Can you work these out from the model? Positions are in its coordinate system, mm. A direction names the side the tool comes from. Coordinates: 2 decimals unless noted, no trailing zeros. Use a Markdown table: item, result. Add a question column.
(1) If I drill on L1, parallel to X at y = -8, z = 11.9; L2, parallel to X at y = -8, z = 11.95; L3, parallel to Y at x = 17, z = 9.25, over which ranges is the centre line in solid material (lowest first)? Write a range as [from, to].
(2) On a 3-axis mill with a long thin cutter (end or side, diameter ignored), from which of +Z, -Z, +X, -X, +Y, -Y can I reach the whole of each face in a straight line? I mean faces 1 (the flat face through (21.38, -5.16, 7.04)), 2 (the flat face through (13, -18, 2)). Say none if no direction works.
(3) We'd pull the mould along X, two halves only. Please class faces 3 (the conical face through (32.351, -32.649, 1.877)), 4 (the cylindrical face through (8.77, 3.44, 6.94)), 5 (the flat face through (20.4, -4.4, 4)), 6 (the flat face through (20.4, -4.4, 10)): pulls with the +X half, pulls with the -X half, needs draft (parallel to the pull), parting line crosses it, or undercut.
(4) I want a section at A-A (z = 9.25). State how many separate pieces and enclosed holes the cut face has, and give its area (3 significant figures).
(5) For pin 1 Ø9.5 at (x, y) = (19, -3) entering from -Z; pin 2 Ø5 at (x, y) = (38.5, -19.5) entering from +Z; pin 3 Ø1 at (y, z) = (-16.5, 9.5) entering from +X; pin 4 Ø7 at (x, y) = (22.5, -12.5) entering from +Z, each with a flat end and sliding along its axis, tell me the tip position at first contact or that it passes through.
```python
from build123d import *

# Parameters (mm, degrees)
BOSS_EXTRUDE1_DEPTH         = 2
BOSS_EXTRUDE2_DEPTH         = 1
CHAMFER1_SIZE               = 0.25
BOSS_EXTRUDE3_DEPTH         = 8
CUT_EXTRUDE_THIN1_START     = -11.887644895
CUT_EXTRUDE_THIN1_OUTLINE_W = 0.5
CUT_EXTRUDE_THIN1_OUTLINE_H = 6
CUT_EXTRUDE_THIN1_DEPTH     = 23
CUT_EXTRUDE1_START          = -0.2
CUT_EXTRUDE1_DEPTH          = 0.2
FILLET1_R                   = 0.1


# Read off the part's stored shape, not the designer's step: Cut-Extrude-Thin1
with BuildPart() as part:
    # Sketch1 → Boss-Extrude1 (new body)
    with BuildSketch(Plane.XY):
        with BuildLine():
            Line((0.767949192, 12), (0.767949192, -48))
            ThreePointArc((0.767949192, -48), (32.790806806, -32.362304412), (45.75, 0.834988321))
            Line((45.75, 0.834988321), (45.75, 12))
            Line((45.75, 12), (0.767949192, 12))
        make_face()
    extrude(amount=BOSS_EXTRUDE1_DEPTH)

    # Sketch2 → Boss-Extrude2 (add)
    with BuildSketch(Plane.XY.offset(2)):
        with BuildLine():
            Line((8.80088089, -1.616278944), (12.994920502, -4.6656628))
            ThreePointArc((12.994920502, -4.6656628), (35.387361749, -15.015949775), (17.487536068, 1.958917118))
            Line((17.487536068, 1.958917118), (13.505420168, 4.854216415))
            ThreePointArc((13.505420168, 4.854216415), (7.91790285, 3.971238374), (8.80088089, -1.616278944))
        make_face()
    boss_extrude2 = extrude(amount=BOSS_EXTRUDE2_DEPTH)

    # Chamfer1
    chamfer1_edges = [part.edges().sort_by_distance(p)[0] for p in [
        (32.790806806, -32.362304412, 2),
        (45.75, 6.41749416, 2),
        (23.258974596, 12, 2),
        (0.767949192, -18, 2),
    ]]
    chamfer(chamfer1_edges, length=CHAMFER1_SIZE)

    # Sketch4 → Boss-Extrude3 (add)
    with BuildSketch(Plane.XY.offset(3)):
        with BuildLine():
            Line((17.520070281, 0.698880903), (12.917352758, 4.045404495))
            ThreePointArc((12.917352758, 4.045404495), (8.726714769, 3.383170965), (9.3889483, -0.807467024))
            Line((9.3889483, -0.807467024), (14.161225934, -4.277273635))
            ThreePointArc((14.161225934, -4.277273635), (34.573815964, -14.433858921), (17.520070281, 0.698880903))
        make_face()
    extrude(amount=BOSS_EXTRUDE3_DEPTH)

    # Mirror1: Boss-Extrude2 across plane
    add(boss_extrude2.mirror(Plane.XY.offset(7)))

    # Cut-Extrude-Thin1 outline → Cut-Extrude-Thin1 (cut)
    with BuildSketch(Plane(origin=(4.627058781, 6.363930791, 0), x_dir=(-0.8088119198432459, 0.5880674096729752, 0), z_dir=(-0.5880674096729752, -0.8088119198432459, 0)).offset(CUT_EXTRUDE_THIN1_START)):
        with Locations((-32.575215368, -7)):
            Rectangle(CUT_EXTRUDE_THIN1_OUTLINE_W, CUT_EXTRUDE_THIN1_OUTLINE_H)
        with Locations((-29.575215368, -7)):
            Rectangle(CUT_EXTRUDE_THIN1_OUTLINE_W, CUT_EXTRUDE_THIN1_OUTLINE_H)
        with Locations((-26.575215368, -7)):
            Rectangle(CUT_EXTRUDE_THIN1_OUTLINE_W, CUT_EXTRUDE_THIN1_OUTLINE_H)
        with Locations((-23.575215368, -7)):
            Rectangle(CUT_EXTRUDE_THIN1_OUTLINE_W, CUT_EXTRUDE_THIN1_OUTLINE_H)
        with Locations((-31.075215368, -7)):
            Rectangle(CUT_EXTRUDE_THIN1_OUTLINE_W, CUT_EXTRUDE_THIN1_OUTLINE_H)
        with Locations((-28.075215368, -7)):
            Rectangle(CUT_EXTRUDE_THIN1_OUTLINE_W, CUT_EXTRUDE_THIN1_OUTLINE_H)
        with Locations((-25.075215368, -7)):
            Rectangle(CUT_EXTRUDE_THIN1_OUTLINE_W, CUT_EXTRUDE_THIN1_OUTLINE_H)
        with Locations((-22.075215368, -7)):
            Rectangle(CUT_EXTRUDE_THIN1_OUTLINE_W, CUT_EXTRUDE_THIN1_OUTLINE_H)
        with Locations((-20.575215368, -7)):
            Rectangle(CUT_EXTRUDE_THIN1_OUTLINE_W, CUT_EXTRUDE_THIN1_OUTLINE_H)
        with Locations((-19.075215368, -7)):
            Rectangle(CUT_EXTRUDE_THIN1_OUTLINE_W, CUT_EXTRUDE_THIN1_OUTLINE_H)
    extrude(amount=CUT_EXTRUDE_THIN1_DEPTH, mode=Mode.SUBTRACT)

    # Sketch9 → Cut-Extrude1 (cut)
    with BuildSketch(Plane.XY.offset(12).offset(CUT_EXTRUDE1_START)):
        with BuildLine():
            Line((17.520070281, 0.698880903), (12.917352758, 4.045404495))
            ThreePointArc((12.917352758, 4.045404495), (8.726714769, 3.383170965), (9.3889483, -0.807467024))
            Line((9.3889483, -0.807467024), (14.161225934, -4.277273635))
            ThreePointArc((14.161225934, -4.277273635), (34.573815964, -14.433858921), (17.520070281, 0.698880903))
        make_face()
    extrude(amount=CUT_EXTRUDE1_DEPTH, mode=Mode.SUBTRACT)

    # Fillet1
    fillet1_edges = [part.edges().sort_by_distance(p)[0] for p in [
        (8.726714769, 3.383170965, 12),
        (11.775087117, -2.542370329, 12),
        (34.573815964, -14.433858921, 12),
        (15.21871152, 2.372142699, 12),
    ]]
    fillet(fillet1_edges, radius=FILLET1_R)


solid = part.part
```
Answers follow:
| question | item | result |
|---|---|---|
| 1 | L1 | x = [12.54, 13.54], [36.54, 37.54] |
| 1 | L2 | x = [12.54, 13.53], [36.56, 37.54] |
| 1 | L3 | y = [-16.22, -14.58], [-13.73, -12.03], [-11.18, -9.48], [-8.63, 1.08] |
| 2 | face 1 | none |
| 2 | face 2 | +Z |
| 3 | face 3 | pulls with the +X half |
| 3 | face 4 | parting line crosses it |
| 3 | face 5 | undercut |
| 3 | face 6 | undercut |
| 4 | separate pieces | 11 |
| 4 | enclosed holes | 0 |
| 4 | area | 357 mm² |
| 5 | pin 1 | stops at z = 0 |
| 5 | pin 2 | stops at z = 2 |
| 5 | pin 3 | stops at x = 33.3 |
| 5 | pin 4 | stops at z = 11.8 |
